The figure shows three views and two pictorial views of one solid part (mm, origin at its lowest corner). Answer the questions. Coordinates: 2 decimals unless noted, no trailing zeros. Loops run counter-clockwise (first coordinate to the right, second up) from the corner with the lowest first, then second, coordinate; pieces in that order, holes last. Notation, with made-up numbers: (-34, 26) -> (11, 26) arc R20 cw to (11, 40) -> close; hole circle Ø2 at (31.5, -8.5). An arc over 180 degrees is marked (long way). Answer as a JSON object with one key per item and string values. Group by question number.
1) Section D-D, the plane y = 7.5 is taken. Give the vertices of the cut face in (x, z), plus the area to 3 significant figures.
2) Section A-A, the plane y = 45 is taken. Give the vertices of the cut face in (x, z).
3) Determine the mould class of the marked faces 1, 2, 3 and 4 for opening direction X: released by +X, released by -X, zero draft, split by the parting line, or undercut.
4) A flat-ended cylindrical pin translates along its axis: P1, Ø3, axis at x = 6.5, y = 5.5, coming from the -Z side. Find the tip coordinate at first contact, or state that the pin passes through.
5) Consider probe 1 along X at (y, z) = (82, 4.5); probe 2 along Z at (x, y) = (9, 34); probe 3 along X at (y, z) = (56, 6.75). Determine where each line is inside the solid, lowest interval first. Write a range as [from, to].
6) Section B-B, the plane z = 10 is taken. Give the vertices of the cut face in (x, y).
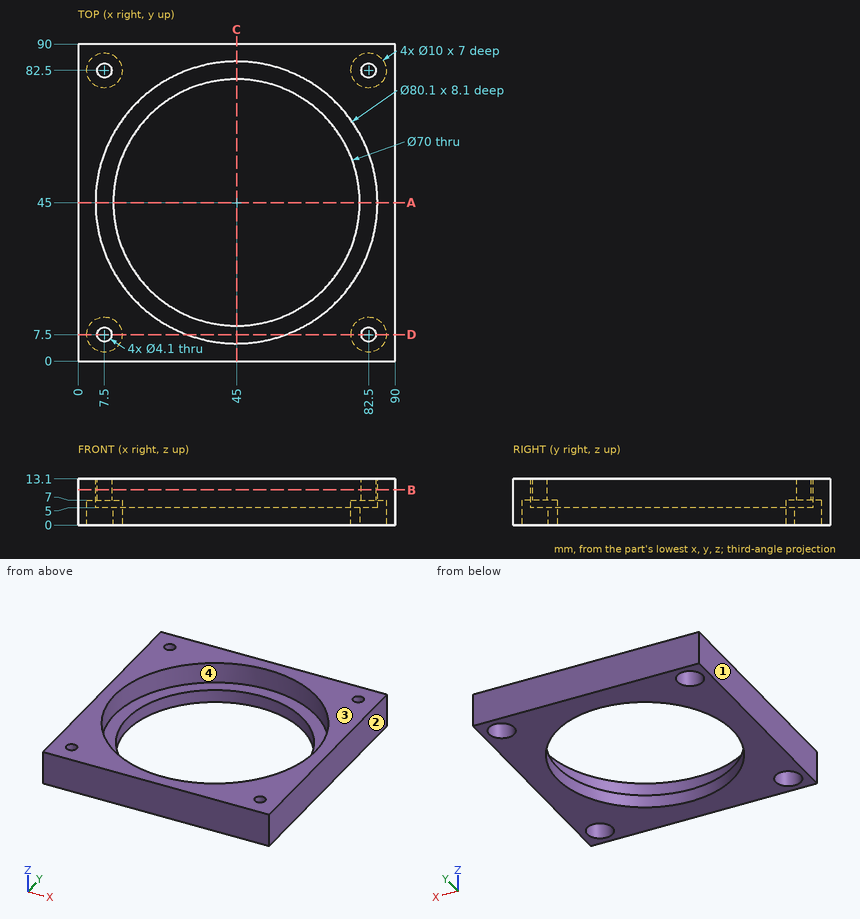
Determined:
{
 "1": {"outline": "(0, 0) -> (2.5, 0) -> (2.5, 7) -> (5.45, 7) -> (5.45, 13.1) -> (0, 13.1) -> close; (9.55, 7) -> (12.5, 7) -> (12.5, 0) -> (77.5, 0) -> (77.5, 7) -> (80.45, 7) -> (80.45, 13.1) -> (59.06, 13.1) -> (59.06, 5) -> (30.94, 5) -> (30.94, 13.1) -> (9.55, 13.1) -> close; (84.55, 7) -> (87.5, 7) -> (87.5, 0) -> (90, 0) -> (90, 13.1) -> (84.55, 13.1) -> close", "area": "761 mm²"},
 "2": {"outline": "(0, 0) -> (10, 0) -> (10, 5) -> (4.95, 5) -> (4.95, 13.1) -> (0, 13.1) -> close; (80, 0) -> (90, 0) -> (90, 13.1) -> (85.05, 13.1) -> (85.05, 5) -> (80, 5) -> close"},
 "3": {"face 1": "released by -X", "face 2": "released by +X", "face 3": "zero draft", "face 4": "undercut"},
 "4": {"P1": "z = 7"},
 "5": {"probe 1": "[0, 2.53], [12.47, 77.53], [87.47, 90]", "probe 2": "[0, 5]", "probe 3": "[0, 6.49], [83.51, 90]"},
 "6": {"outline": "(0, 0) -> (90, 0) -> (90, 90) -> (0, 90) -> close; hole circle Ø80.1 at (45, 45); hole circle Ø4.1 at (7.5, 7.5); hole circle Ø4.1 at (7.5, 82.5); hole circle Ø4.1 at (82.5, 7.5); hole circle Ø4.1 at (82.5, 82.5)"}
}
